```python
from build123d import *

# Parameters (mm, degrees)
SKETCH_1_R               = 3
EXTRUDE_1_DEPTH          = 5
CHAMFER_1_SIZE           = 0.5
SKETCH_2_R               = 2
CUT_EXTRUDE_1_DEPTH      = 1
CUT_EXTRUDE_1_DEPTH_BACK = 6
CHAMFER_2_SIZE           = 0.5


with BuildPart() as part:
    # 草图1 → 凸台-拉伸1 (new body)
    with BuildSketch(Plane.XY):
        with BuildLine():
            ThreePointArc((-56.275757576, -7.325223765), (-60.374306352, 3.240512704), (-49.794769231, 7.303305281))
            ThreePointArc((-49.794769231, 7.303305281), (-26.53, 2.339355406), (-3.265230769, 7.303305281))
            ThreePointArc((-3.265230769, 7.303305281), (7.314306352, 3.240512704), (3.215757576, -7.325223765))
            ThreePointArc((3.215757576, -7.325223765), (-26.53, -13.566903935), (-56.275757576, -7.325223765))
        make_face()
        Circle(SKETCH_1_R, mode=Mode.SUBTRACT)
        with Locations((-53.06, 0)):
            Circle(SKETCH_1_R, mode=Mode.SUBTRACT)
    extrude(amount=EXTRUDE_1_DEPTH)

    # 倒角1
    chamfer_1_edges = [part.edges().sort_by_distance(p)[0] for p in [
        (-3, 0, 0),
        (-3, 0, 5),
        (-26.53, 2.339355406, 5),
        (-56.06, 0, 0),
        (-56.06, 0, 5),
        (-60.374306352, 3.240512704, 5),
        (-26.53, -13.566903935, 5),
        (-60.374306352, 3.240512704, 0),
        (-26.53, 2.339355406, 0),
        (7.314306352, 3.240512704, 0),
        (-26.53, -13.566903935, 0),
        (7.314306352, 3.240512704, 5),
    ]]
    chamfer(chamfer_1_edges, length=CHAMFER_1_SIZE)

    # 草图2 → 切除-拉伸1 (cut, two sides)
    with BuildSketch(Plane(origin=(0, 0, 0), x_dir=(-1, 0, 0), z_dir=(0, 0, -1))) as cut_extrude_1_sk:
        with Locations((10.396009946, -3.594854266)):
            Circle(SKETCH_2_R)
    extrude(amount=CUT_EXTRUDE_1_DEPTH, mode=Mode.SUBTRACT)
    extrude(cut_extrude_1_sk.sketch, amount=-CUT_EXTRUDE_1_DEPTH_BACK, mode=Mode.SUBTRACT)

    # 倒角2
    chamfer_2_edges = [part.edges().sort_by_distance(p)[0] for p in [
        (-8.396009946, -3.594854266, 5),
        (-8.396009946, -3.594854266, 0),
    ]]
    chamfer(chamfer_2_edges, length=CHAMFER_2_SIZE)


solid = part.part
```
Geometry: final body of the model. Coordinates: model frame, mm. Coordinates: 2 decimals unless noted, no trailing zeros. Order: outer loops, then holes, each group sorted by start corner. A loop starts at its lowest first (then second) coordinate and runs counter-clockwise, first axis right, second up. Notation, with made-up numbers: (45, 74) -> (94, 74) arc R27 ccw to (94, 99) -> close; hole circle Ø5 at (-35.75, 62). An arc over 180 degrees is marked (long way). Write item = value, one per line.
(1) Cut plane A-A on y = 0. Return loops of the section in (x, z), plus the area to 3 significant figures.
Solved:
outline = (-61.06, 0.5) -> (-60.56, 0) -> (-56.56, 0) -> (-56.06, 0.5) -> (-56.06, 4.5) -> (-56.56, 5) -> (-60.56, 5) -> (-61.06, 4.5) -> close; (-50.06, 0.5) -> (-49.56, 0) -> (-3.5, 0) -> (-3, 0.5) -> (-3, 4.5) -> (-3.5, 5) -> (-49.56, 5) -> (-50.06, 4.5) -> close; (3, 0.5) -> (3.5, 0) -> (7.5, 0) -> (8, 0.5) -> (8, 4.5) -> (7.5, 5) -> (3.5, 5) -> (3, 4.5) -> close
area = 284 mm²
(2) Line query: line 1 (X direction, y = -0.25, z = 4.3); line 2 (X direction, y = 1.5, z = 4.7); line 3 (X direction, y = -2, z = 4). Output: solid intervals per line, ascending.
Solved:
line_1 = -61.06 to -56.05, -50.07 to -2.99, 2.99 to 8
line_2 = -60.71 to -55.89, -50.23 to -2.83, 2.83 to 7.65
line_3 = -60.81 to -55.3, -50.82 to -11.6, -9.19 to -2.24, 2.24 to 7.75
(3) Pull-direction query (Y, two-part tool) for faces 1 (the cylindrical face through (-56.057, 0.132, 2.472)), 2 (the cylindrical face through (-26.101, -13.566, 2.472)), 3 (the cylindrical face through (-26.87, 2.34, 2.47)); classes: pulls with the +Y half, pulls with the -Y half, needs draft (parallel to the pull), parting line crosses it, or undercut.
Solved:
face_1 = undercut
face_2 = pulls with the -Y half
face_3 = pulls with the +Y half
(4) Pin query (flat end, axial travel): pin 1 Ø9.5 at (x, y) = (-53.06, 0) entering from +Z; pin 2 Ø2 at (y, z) = (5, 1.5) entering from +X. Return the tip coordinate at first contact, or that it passes through.
Solved:
pin_1 = 5
pin_2 = 6.93
(5) Cut plane B-B on z = 2.6. Return loops of the section in (x, y), plus the area to 3 significant figures.
Solved:
outline = (-56.28, -7.33) arc R74 ccw to (3.22, -7.33) arc R8 ccw (long way) to (-3.27, 7.3) arc R57 cw to (-49.79, 7.3) arc R8 ccw (long way) to start; hole circle Ø6 at (-53.06, 0); hole circle Ø4 at (-10.4, -3.59); hole circle Ø6 at (0, 0)
area = 1,000 mm²
